Design review of the part built by this model. Coordinates are the model's own, in mm. Coordinates: 2 decimals unless noted, no trailing zeros. Loops run counter-clockwise (first coordinate to the right, second up) from the corner with the lowest first, then second, coordinate; pieces in that order, holes last. Notation, with made-up numbers: (11, 82.5) - (64, 82.5) arc R9 cw to (64, 87.5) - close; hole circle Ø6 at (-25, 35.25). An arc over 180 degrees is marked (long way). Answer in a Markdown table with one row per item. Add a question column.
(1) Clearance check with a flat-ended pin moving along its axis: pin 1 (8 mm diameter, centred on y = 100, z = 105.5, fed in from +X). State where the tip first meets the part, or that it passes through.
(2) We need section C-C, the plane y = 82. Write out the cut boundary in (x, z), plus the area to 3 significant figures.
(3) We need section B-B, the plane x = 118.5. Write out the cut boundary in (y, z), plus the area to 3 significant figures.
(4) We need section A-A, the plane z = 104. Write out the cut boundary in (x, y).
(5) To check wall thickness, follow L1, parallel to Y at x = 118.75, z = 91.5; L2, parallel to Z at x = 118.55, y = 69; L3, parallel to Y at x = 118.65, z = 110.5. State the ranges of each line that lie inside material, in increasing order. Write a range as [from, to].
from build123d import *

# Parameters (mm, degrees)
BOX056_W     = 5
BOX056_H     = 58
BOX056_DEPTH = 25
FILLET062_R  = 2.5
BOX007_W     = 1
BOX007_H     = 60
BOX007_DEPTH = 27
FILLET045_R  = 3


with BuildPart() as fillet062:
    # Box056 → Box056 (new body)
    with BuildSketch(Plane(origin=(118, 56, 86), x_dir=(1, 0, 0), z_dir=(0, 0, 1))):
        with Locations((2.5, 29)):
            Rectangle(BOX056_W, BOX056_H)
    extrude(amount=BOX056_DEPTH)

    # Fillet062
    fillet062_edges = [fillet062.edges().sort_by_distance(p)[0] for p in [
        (120.5, 56, 86),
        (120.5, 56, 111),
        (120.5, 114, 86),
        (120.5, 114, 111),
    ]]
    fillet(fillet062_edges, radius=FILLET062_R)


with BuildPart() as cut042:
    # Box007 → Box007 (new body)
    with BuildSketch(Plane(origin=(118, 55, 85), x_dir=(1, 0, 0), z_dir=(0, 0, 1))):
        with Locations((0.5, 30)):
            Rectangle(BOX007_W, BOX007_H)
    extrude(amount=BOX007_DEPTH)

    # Fillet045
    fillet045_edges = [cut042.edges().sort_by_distance(p)[0] for p in [
        (118.5, 55, 85),
        (118.5, 55, 112),
        (118.5, 115, 85),
        (118.5, 115, 112),
    ]]
    fillet(fillet045_edges, radius=FILLET045_R)

    # Cut042: cut Fillet062
    add(fillet062.part, mode=Mode.SUBTRACT)


solid = cut042.part
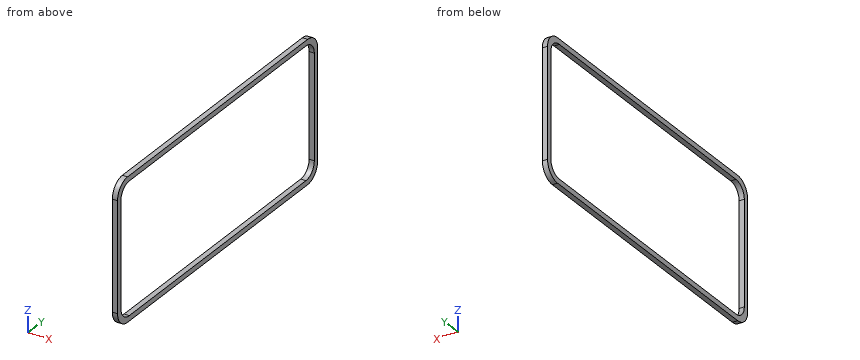
Responses:
| question | item | result |
|---|---|---|
| 1 | pin 1 | passes through |
| 2 | outline | (118, 85) - (119, 85) - (119, 86) - (118, 86) - close; (118, 111) - (119, 111) - (119, 112) - (118, 112) - close |
| 2 | area | 2.00 mm2 |
| 3 | outline | (55, 88) arc R3 ccw to (58, 85) - (112, 85) arc R3 ccw to (115, 88) - (115, 109) arc R3 ccw to (112, 112) - (58, 112) arc R3 ccw to (55, 109) - close; hole (56, 88.5) arc R2.5 ccw to (58.5, 86) - (111.5, 86) arc R2.5 ccw to (114, 88.5) - (114, 108.5) arc R2.5 ccw to (111.5, 111) - (58.5, 111) arc R2.5 ccw to (56, 108.5) - close |
| 3 | area | 168 mm2 |
| 4 | outline | (118, 55) - (119, 55) - (119, 56) - (118, 56) - close; (118, 114) - (119, 114) - (119, 115) - (118, 115) - close |
| 5 | L1 | y = [55, 56], [114, 115] |
| 5 | L2 | z = [85, 86], [111, 112] |
| 5 | L3 | y = [55.4, 57], [113, 114.6] |
